```python
from build123d import *

# Parameters (mm, degrees)
SKETCH1_W                                  = 290
SKETCH1_H                                  = 212
BOSS_EXTRUDE1_DEPTH                        = 10
SKETCH2_W                                  = 290
SKETCH2_H                                  = 212
SKETCH2_W_2                                = 282
SKETCH2_H_2                                = 202
BOSS_EXTRUDE2_DEPTH                        = 70
SKETCH3_W                                  = 6
SKETCH3_H                                  = 202
SKETCH3_W_2                                = 40
SKETCH3_H_2                                = 40
SKETCH3_W_3                                = 30
SKETCH3_H_3                                = 30
BOSS_EXTRUDE3_DEPTH                        = 10
CHAMFER1_SIZE                              = 10
SKETCH4_R                                  = 2.5
CUT_EXTRUDE1_DEPTH                         = 207
SKETCH5_R                                  = 2.5
CUT_EXTRUDE2_DEPTH                         = 270.014869478
MIRROR2_AT_THE_SECOND_PLANE_COPY_1_SKETC_R = 2.5
MIRROR2_AT_THE_SECOND_PLANE_COPY_1_DEPTH   = 207


with BuildPart() as part:
    # Sketch1 → Boss-Extrude1 (new body)
    with BuildSketch(Plane(origin=(0, 0, 0), x_dir=(1, 0, 0), z_dir=(0, 1, 0))):
        Rectangle(SKETCH1_W, SKETCH1_H)
    extrude(amount=BOSS_EXTRUDE1_DEPTH)

    # Sketch2 → Boss-Extrude2 (add)
    with BuildSketch(Plane(origin=(0, 10, 0), x_dir=(1, 0, 0), z_dir=(0, 1, 0))):
        Rectangle(SKETCH2_W, SKETCH2_H)
        Rectangle(SKETCH2_W_2, SKETCH2_H_2, mode=Mode.SUBTRACT)
    extrude(amount=BOSS_EXTRUDE2_DEPTH)

    # Sketch3 → Boss-Extrude3 (add)
    # profile 1 of 2: a face of its own
    with BuildSketch(Plane(origin=(0, 10, 0), x_dir=(1, 0, 0), z_dir=(0, 1, 0))):
        with Locations((138, 0)):
            Rectangle(SKETCH3_W, SKETCH3_H)
    # profile 2 of 2: a face of its own
    with BuildSketch(Plane(origin=(0, 10, 0), x_dir=(1, 0, 0), z_dir=(0, 1, 0))):
        Rectangle(SKETCH3_W_2, SKETCH3_H_2)
        Rectangle(SKETCH3_W_3, SKETCH3_H_3, mode=Mode.SUBTRACT)
    extrude(amount=BOSS_EXTRUDE3_DEPTH)

    # Chamfer1
    chamfer1_edges = [part.edges().sort_by_distance(p)[0] for p in [
        (0, 0, 106),
        (-145, 0, 0),
        (0, 0, -106),
        (145, 0, 0),
    ]]
    chamfer(chamfer1_edges, length=CHAMFER1_SIZE)

    # Sketch4 → Cut-Extrude1 (cut)
    with BuildSketch(Plane.XY.offset(106)):
        with Locations((-44.6, 30)):
            Circle(SKETCH4_R)
        with Locations((-74.6, 30)):
            Circle(SKETCH4_R)
        with Locations((-59.6, 70)):
            Circle(SKETCH4_R)
    cut_extrude1 = extrude(amount=-CUT_EXTRUDE1_DEPTH, mode=Mode.SUBTRACT)

    # Sketch5 → Cut-Extrude2 (cut, through all)
    with BuildSketch(Plane.XY.offset(106)):
        with Locations((-130, 70)):
            Circle(SKETCH5_R)
        with Locations((-130, 30)):
            Circle(SKETCH5_R)
        with Locations((-110, 40)):
            Circle(SKETCH5_R)
    cut_extrude2 = extrude(amount=-CUT_EXTRUDE2_DEPTH, mode=Mode.SUBTRACT)

    # Mirror1: Cut-Extrude2 across plane
    add(cut_extrude2.mirror(Plane(origin=(0, 0, 0), x_dir=(0, 0, 1), z_dir=(1, 0, 0))), mode=Mode.SUBTRACT)

    # Mirror2: Cut-Extrude1 across plane
    add(cut_extrude1.mirror(Plane(origin=(0, 0, 0), x_dir=(0, 0, 1), z_dir=(1, 0, 0))), mode=Mode.SUBTRACT)

    # Mirror2 at the second plane: Cut-Extrude1 across plane
    add(cut_extrude1.mirror(Plane.XY), mode=Mode.SUBTRACT)

    # Mirror2 at the second plane copy 1 sketc → Mirror2 at the second plane copy 1 (cut)
    with BuildSketch(Plane(origin=(0, 0, -106), x_dir=(-1, 0, 0), z_dir=(0, 0, -1))):
        with Locations((-44.6, 30)):
            Circle(MIRROR2_AT_THE_SECOND_PLANE_COPY_1_SKETC_R)
        with Locations((-74.6, 30)):
            Circle(MIRROR2_AT_THE_SECOND_PLANE_COPY_1_SKETC_R)
        with Locations((-59.6, 70)):
            Circle(MIRROR2_AT_THE_SECOND_PLANE_COPY_1_SKETC_R)
    extrude(amount=-MIRROR2_AT_THE_SECOND_PLANE_COPY_1_DEPTH, mode=Mode.SUBTRACT)


solid = part.part
```
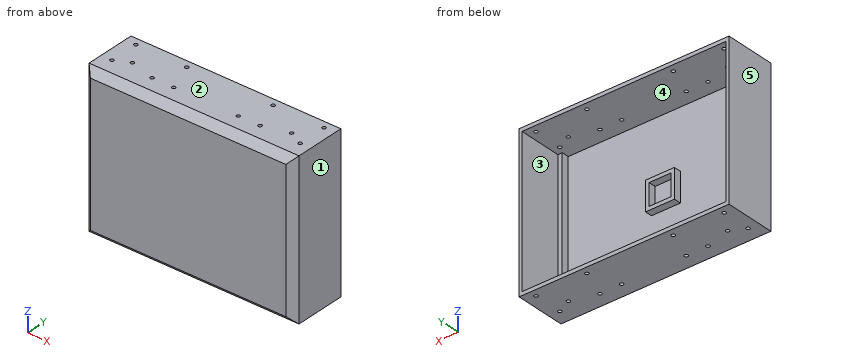
The listing builds one solid part. Answer for the finished solid, in the listing's coordinates (mm). Face numbers are marked on the shaded views. A direction names the side the tool comes from. Give positions to 0.01 mm unless a question says otherwise; leave off trailing zeros. Order: outer loops, then holes, each group sorted by start corner. A loop starts at its lowest first (then second) coordinate and runs counter-clockwise, first axis right, second up. Notation, with made-up numbers: M -34,30.25 L -25,30.25 A27 ccw -25,59.25 Z; hole C -14.75,-19 d7. An arc over 180 degrees is marked long. Put each result on its own line as item: value. Start each with the question number.
Item 1: The part is cut by section C-C, the plane x = -27.5. Determine the outline of the cut face in (y, z).
Item 2: The part is cut by section A-A, the plane z = 8. Determine the outline of the cut face in (x, y), and give its area (3 significant figures).
Item 3: Flat-ended cylindrical pins translate along their axes: P1, Ø12, axis at x = -94.5, z = 62, coming from the +Y side; P2, Ø4.5, axis at x = 130, y = 30, coming from the +Z side. Find the tip coordinate at first contact, or state that the pin passes through.
Item 4: For a pull along Z with two mould halves and no side action, classify the marked faces 1, 2 and 3 as +Z half, -Z half, draft (parallel to the pull), parting line (faces both ways), or undercut.
Item 5: The part is cut by section D-D, the plane z = 34. Determine the outline of the cut face in (x, y), and give its area (3 significant figures).
Item 6: The part is cut by section B-B, the plane y = 24. Determine the outline of the cut face in (x, z), and give its area (3 significant figures).
Item 7: Find the intervals of material crossed by line 1 along X through (y, z) = (68, 96); line 2 along Z through (x, y) = (80.5, 21); line 3 along X through (y, z) = (12, -0.5), in increasing order.
Item 8: Which of the six approach directions +Z, -Z, +X, -X, +Y, -Y give full straight-line access (tool end or side, diameter ignored) to the marked faces 4 and 5?
Answer key:
1. outline: M 0,-96 L 10,-106 L 80,-106 L 80,-101 L 10,-101 L 10,101 L 80,101 L 80,106 L 10,106 L 0,96 Z
2. outline: M -145,10 L -135,0 L 135,0 L 145,10 L 145,80 L 141,80 L 141,20 L 135,20 L 135,10 L 20,10 L 20,20 L 15,20 L 15,10 L -15,10 L -15,20 L -20,20 L -20,10 L -141,10 L -141,80 L -145,80 Z
2. area: 3,520 mm²
3. P1: stops at y = 10
3. P2: passes through
4. face 1: draft
4. face 2: +Z half
4. face 3: undercut
5. outline: M -145,10 L -135,0 L 135,0 L 145,10 L 145,80 L 141,80 L 141,20 L 135,20 L 135,10 L -141,10 L -141,80 L -145,80 Z
5. area: 3,420 mm²
6. outline: M -145,-106 L 145,-106 L 145,106 L -145,106 Z; hole M -141,-101 L 141,-101 L 141,101 L -141,101 Z
6. area: 4,520 mm²
7. line 1: x = -145 to -141, 141 to 145
7. line 2: z = -106 to -101, 101 to 106
7. line 3: x = -145 to -141, -20 to -15, 15 to 20, 135 to 145
8. face 4: +Y
8. face 5: +Z, -Z, -X, +Y, -Y
